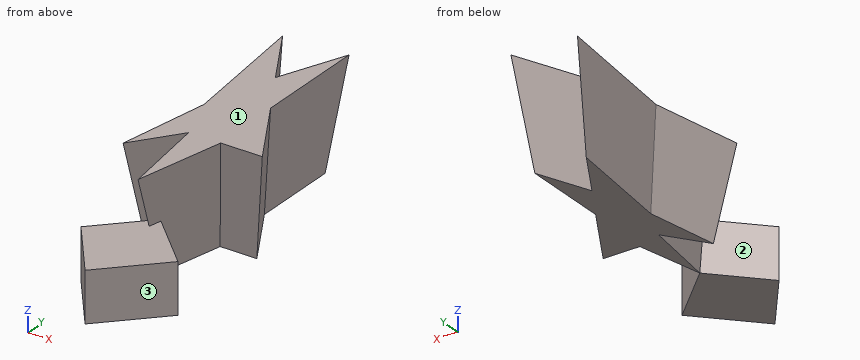
from build123d import *

# Parameters (mm, degrees)
F1_DEPTH = 50.8
F1_TAPER = -3
F3_DEPTH = 25.4


with BuildPart() as f1:
    # F0 (on Top) → F1 (new body)
    with BuildSketch(Plane.XY):
        Polygon((-5.1951231435, 37.5182926655), (0, 0), (7.1364506148, 33.4682352841), (25.7764216512, 33.4682352841), (6.0908943415, 67.2407448292), (6.0908943415, 111.572496593), (-4.6124211513, 85.2674916387), (-19.497255753, 110.8039281665), (-13.200096786, 54.7134391963), (-19.497255753, 18.1095562875), align=None)
    extrude(amount=F1_DEPTH, taper=F1_TAPER)

    # F2 (on Top) → F3 (join)
    with BuildSketch(Plane.XY):
        Polygon((27.3833926767, -26.3573322445), (0, 0), (-23.3508690358, -24.2598913356), (0, -54.8067286982), align=None)
    extrude(amount=F3_DEPTH)


solid = f1.part
The listing builds one solid part. Answer for the finished solid, in the listing's coordinates (mm). Face numbers are marked on the shaded views. Coordinates: 2 decimals unless noted, no trailing zeros. Loops run counter-clockwise (first coordinate to the right, second up) from the corner with the lowest first, then second, coordinate; pieces in that order, holes last. Notation, with made-up numbers: (84.5, -13.75) -> (107.5, -13.75) arc R34 cw to (107.5, 23.25) -> close; hole circle Ø9 at (4.25, 57.25). An arc over 180 degrees is marked (long way). Write item = value, one per line. Start each with the question number.
1) The mould has two halves that part along X. Classify the marked faces 1, 2 and 3: released by +X, released by -X, zero draft, split by the parting line, or undercut.
2) Given pin 1 Ø4 at (x, y) = (-4, -6.5) entering from +Z; pin 2 Ø1.5 at (x, z) = (3, 11) entering from -Y; pin 3 Ø2 at (x, z) = (9, 15) entering from +Y, each flat-ended and moving along its own axis, determine where each tip first touches the part or whether it passes through.
3) Straight lines are drawn through the part: line 1 (X direction, y = 102, z = 43.5); line 2 (X direction, y = 26, z = 40); line 3 (Y direction, x = -8, z = 7). For each, find the intervals that lie inside material, in ascending order. Write a range as from..to.
4) A cutting plane is placed at A-A (y = -35.5). Give the vertices of the cut face in (x, z), then the cut area to 3 significant figures.
Responses:
q1.face_1 = zero draft
q1.face_2 = released by -X
q1.face_3 = released by +X
q2.pin_1 = 25.4
q2.pin_2 = -52.47
q2.pin_3 = 65.53
q3.line_1 = -20.8..-11.73, -0.27..8.37
q3.line_2 = -20.27..-11.08, -5.72..7.69
q3.line_3 = -44.34..-8.31, 33.09..91.81
q4.outline = (-14.76, 0) -> (18.58, 0) -> (18.58, 25.4) -> (-14.76, 25.4) -> close
q4.area = 847 mm²
